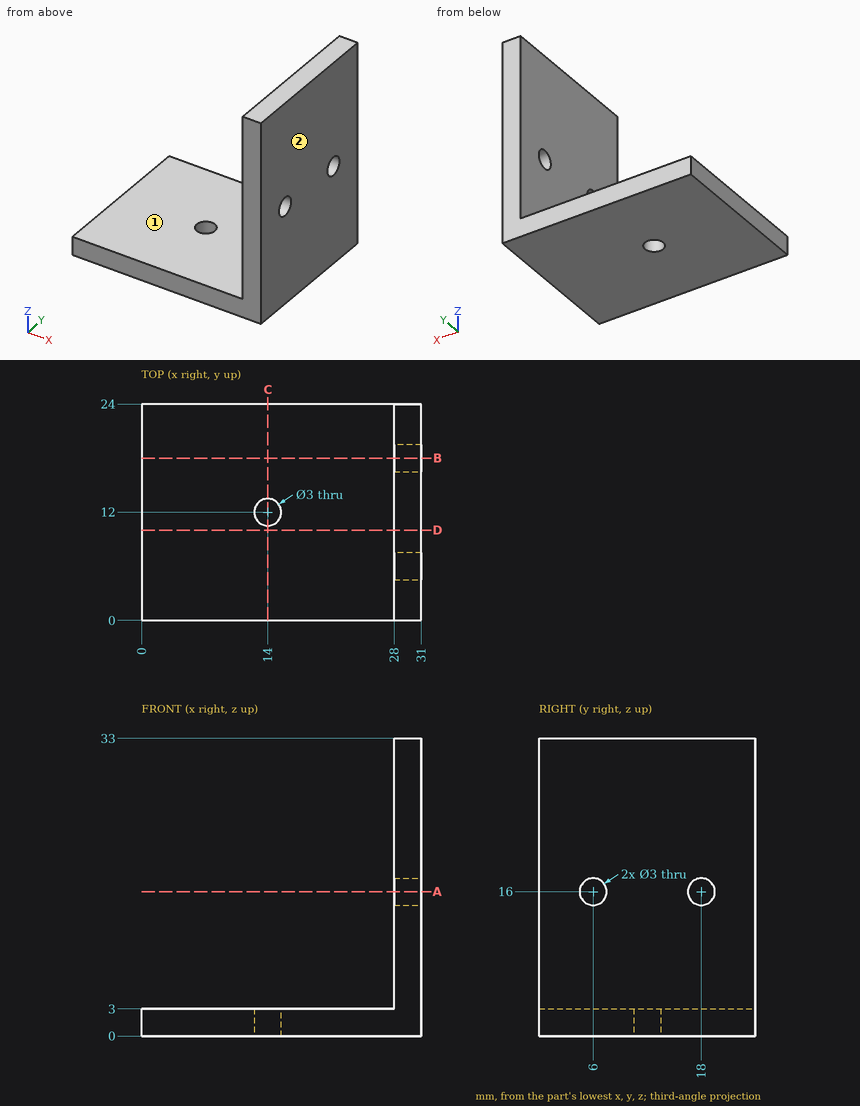
Design review of the part shown in the three views and the two pictorial views. Dimensions are in mm from the part's minimum x, y and z. A direction names the side the tool comes from. Round coordinates to 2 decimals unless told otherwise and drop trailing zeros. Loops run counter-clockwise (first coordinate to the right, second up) from the corner with the lowest first, then second, coordinate; pieces in that order, holes last. Notation, with made-up numbers: (29.25, -33) -> (61.25, -33) arc R20 cw to (61.25, -8) -> close; hole circle Ø4 at (9, 46). An arc over 180 degrees is marked (long way). Use one line per item in the form item = value. Start each with the question number.
Q1. Wall thickness on line 1 along Z through (x, y) = (29.95, 6); line 2 along Y through (x, z) = (14, 2); line 3 along Z through (x, y) = (4.5, 6.25): over which ranges is each line inside the solid? List them lowest first. Write a range as [from, to].
Q2. We need section D-D on y = 10. Give the boundary of the cut face in (x, z).
Q3. We need section B-B on y = 18. Give the boundary of the cut face in (x, z), then the cut area to 3 significant figures.
Q4. Machinability: for the marked faces 1 and 2, which of the approach directions +Z, -Z, +X, -X, +Y, -Y give a long, thin tool a straight path to every point of the face, cutting with its end or side? Answer none if there is none.
Q5. For pin 1 Ø7 at (y, z) = (8.5, 20.5) entering from -X; pin 2 Ø12 at (x, y) = (12, 4) entering from +Z, all flat-tipped, find the tip position at first contact; note any pin that passes through.
Q6. We need section C-C on x = 14. Give the boundary of the cut face in (y, z).
Q7. We need section A-A on z = 16. Give the boundary of the cut face in (x, y).
Calculated:
q1.line_1 = [0, 14.5], [17.5, 33]
q1.line_2 = [0, 10.5], [13.5, 24]
q1.line_3 = [0, 3]
q2.outline = (0, 0) -> (31, 0) -> (31, 33) -> (28, 33) -> (28, 3) -> (0, 3) -> close
q3.outline = (0, 0) -> (31, 0) -> (31, 14.5) -> (28, 14.5) -> (28, 3) -> (0, 3) -> close; (28, 17.5) -> (31, 17.5) -> (31, 33) -> (28, 33) -> close
q3.area = 174 mm²
q4.face_1 = +Z, -X, +Y, -Y
q4.face_2 = +Z, -Z, +X, +Y, -Y
q5.pin_1 = 28
q5.pin_2 = 3
q6.outline = (0, 0) -> (10.5, 0) -> (10.5, 3) -> (0, 3) -> close; (13.5, 0) -> (24, 0) -> (24, 3) -> (13.5, 3) -> close
q7.outline = (28, 0) -> (31, 0) -> (31, 4.5) -> (28, 4.5) -> close; (28, 7.5) -> (31, 7.5) -> (31, 16.5) -> (28, 16.5) -> close; (28, 19.5) -> (31, 19.5) -> (31, 24) -> (28, 24) -> close
